```python
from build123d import *

# Parameters (mm, degrees)
SALIENTE_EXTRUIR1_DEPTH      = 60
CORTAR_EXTRUIR1_DEPTH        = 30
SALIENTE_EXTRUIR2_REACH      = 216.709
SALIENTE_EXTRUIR2_END_RADIUS = 50
CROQUIS3_R                   = 50


with BuildPart() as part:
    # Croquis1 → Saliente-Extruir1 (new, symmetric)
    with BuildSketch(Plane(origin=(0, 0, 0), x_dir=(0, 0, -1), z_dir=(1, 0, 0))):
        with BuildLine():
            Line((-50, 80), (-50, 0))
            ThreePointArc((-50, 0), (0, -50), (50, 0))
            Line((50, 0), (50, 80))
            ThreePointArc((50, 80), (0, 130), (-50, 80))
        make_face()
    extrude(amount=SALIENTE_EXTRUIR1_DEPTH, both=True)

    # Croquis2 → Cortar-Extruir1 (cut, symmetric)
    with BuildSketch(Plane(origin=(0, 0, 0), x_dir=(0, 0, -1), z_dir=(1, 0, 0))):
        with BuildLine():
            Line((-50, 70), (50, 70))
            Line((50, 70), (50, 0))
            ThreePointArc((50, 0), (0, -50), (-50, 0))
            Line((-50, 0), (-50, 70))
        make_face()
    extrude(amount=CORTAR_EXTRUIR1_DEPTH, both=True, mode=Mode.SUBTRACT)

    # Saliente-Extruir2: up to this cylinder (the profile starts outside it)
    saliente_extruir2_end = Plane(origin=(0, 80, 0), z_dir=(-1, 0, 0)) * Cylinder(SALIENTE_EXTRUIR2_END_RADIUS, 534.418, mode=Mode.PRIVATE)
    # Croquis3 → Saliente-Extruir2 (add, up to the surface)
    with BuildSketch(Plane(origin=(0, 150, 0), x_dir=(1, 0, 0), z_dir=(0, 1, 0)), mode=Mode.PRIVATE) as saliente_extruir2_sk1:
        with Locations(Location((0, 0, 0), (0, 0, 270))):
            Circle(CROQUIS3_R)
    saliente_extruir2_tool1 = extrude(saliente_extruir2_sk1.sketch, amount=-SALIENTE_EXTRUIR2_REACH, mode=Mode.PRIVATE) - saliente_extruir2_end
    add(saliente_extruir2_tool1.solids().sort_by_distance((0, 150, 0))[0])


solid = part.part
```
Geometry check sheet. Reference: the model listing, model coordinates, mm. A direction names the side the tool comes from. Round coordinates to 2 decimals unless told otherwise and drop trailing zeros. Loops run counter-clockwise (first coordinate to the right, second up) from the corner with the lowest first, then second, coordinate; pieces in that order, holes last. Notation, with made-up numbers: (22, 13) - (50, 13) arc R16 cw to (50, 20) - close; hole circle Ø8 at (-21.75, 47). An arc over 180 degrees is marked (long way). Write each question's results on one line, items separated by ' | '. Start each with the question number.
Q1. Release check for a two-part mould opening along X. For faces 5 (the flat face through (1, 75, -50)), 6 (the flat face through (0, 70, 1)), 7 (the flat face through (60, 41, 1)) record: +X half, -X half, draft (parallel to the pull), parting line (faces both ways), or undercut.
Q2. Cross-section at C-C on x = 39. Enter the section's corners in (y, z).
Q3. Thickness scan on line 1 (X direction, y = 63, z = -2); line 2 (Z direction, x = -43.5, y = 120); line 3 (Y direction, x = -12, z = 35). Record the ranges inside material, lowest first. Write a range as [from, to].
Q4. Cross-section at B-B on z = 0. Enter the section's corners in (x, y), and give its area (3 significant figures).
Q5. Cross-section at D-D on y = -25.5. Enter the section's corners in (x, z), and give its area (3 significant figures).
Q6. Cross-section at A-A on y = 65. Enter the section's corners in (x, z).
Q7. Gauge pin test, flat ends, axial feed: P1, Ø10, axis at x = -28, z = 4.5, coming from the -Y side; P2, Ø1.5, axis at x = 17.5, z = -30, coming from the -Y side; P3, Ø1.5, axis at x = -4.5, y = 124, coming from the +Z side. Record the tip position at first contact, or that the pin passes through.
Q8. Access from +Z, -Z, +X, -X, +Y, -Y to the whole of each face (thin tool, end or side, straight path). Record for faces 1 (the cylindrical face through (-49.58, 126.597, -18.13)), 2 (the flat face through (30, 11, -1)), 3 (the cylindrical face through (50.42, 129.988, -1.099)), 4 (the cylindrical face through (33.792, 131.046, -36.852)).
Answers below:
1) face 5: draft | face 6: undercut | face 7: +X half
2) outline: (0, -50) - (80, -50) arc R50 ccw to (119, -31.29) - (150, -31.29) - (150, 31.29) - (119, 31.29) arc R50 ccw to (80, 50) - (0, 50) arc R50 ccw to start
3) line 1: x = [-60, -30], [30, 60] | line 2: z = [-30, 30] | line 3: y = [70, 150]
4) outline: (-60, -50) - (-30, -50) - (-30, 70) - (30, 70) - (30, -50) - (60, -50) - (60, 130) - (50, 130) - (50, 150) - (-50, 150) - (-50, 130) - (-60, 130) - close | area: 16,400 mm²
5) outline: (-60, -43.01) - (-30, -43.01) - (-30, 43.01) - (-60, 43.01) - close; (30, -43.01) - (60, -43.01) - (60, 43.01) - (30, 43.01) - close | area: 5,160 mm²
6) outline: (-60, -50) - (-30, -50) - (-30, 50) - (-60, 50) - close; (30, -50) - (60, -50) - (60, 50) - (30, 50) - close
7) P1: stops at y = -50 | P2: stops at y = 70 | P3: stops at z = 49.86
8) face 1: -X, +Y | face 2: +Z, -Z, -Y | face 3: +X, +Y | face 4: +Y
